from build123d import *

# Parameters (mm, degrees)
SKETCH1_W               = 270
SKETCH1_H               = 100
BOSS_EXTRUDE1_DEPTH     = 3.175
SKETCH1_H_2             = 140
BOSS_EXTRUDE1_2_DEPTH   = 3.175
SKETCH2_R               = 2.5
CUT_EXTRUDE1_DEPTH      = 1
CUT_EXTRUDE1_DEPTH_BACK = 4.175


with BuildPart() as part:
    # Sketch1 → Boss-Extrude1 (new body)
    with BuildSketch(Plane(origin=(0, 0, 0), x_dir=(1, 0, 0), z_dir=(0, 1, 0))):
        with Locations((135, 50)):
            Rectangle(SKETCH1_W, SKETCH1_H)
    extrude(amount=BOSS_EXTRUDE1_DEPTH)


with BuildPart() as body_2:
    # Sketch1 → Boss-Extrude1 2 (new body)
    with BuildSketch(Plane(origin=(0, 0, 0), x_dir=(1, 0, 0), z_dir=(0, 1, 0))):
        with Locations((135, 175)):
            Rectangle(SKETCH1_W, SKETCH1_H_2)
    extrude(amount=BOSS_EXTRUDE1_2_DEPTH)


with BuildPart() as cut_extrude1_tool:
    # Sketch2 → Cut-Extrude1 (new body, two sides)
    with BuildSketch(Plane(origin=(0, 3.175, 0), x_dir=(1, 0, 0), z_dir=(0, 1, 0))) as cut_extrude1_sk:
        with Locations((10, 175)):
            Circle(SKETCH2_R)
        with Locations((10, 50)):
            Circle(SKETCH2_R)
        with Locations((260, 50)):
            Circle(SKETCH2_R)
        with Locations((260, 175)):
            Circle(SKETCH2_R)
        with Locations((135, 115)):
            Circle(SKETCH2_R)
        with Locations((135, 235)):
            Circle(SKETCH2_R)
        with Locations((135, 90)):
            Circle(SKETCH2_R)
        with Locations((135, 10)):
            Circle(SKETCH2_R)
        with BuildLine():
            Line((117.5, 79), (152.5, 79))
            ThreePointArc((152.5, 79), (156.5, 75), (152.5, 71))
            Line((152.5, 71), (117.5, 71))
            ThreePointArc((117.5, 71), (113.5, 75), (117.5, 79))
        make_face()
    extrude(amount=CUT_EXTRUDE1_DEPTH)
    extrude(cut_extrude1_sk.sketch, amount=-CUT_EXTRUDE1_DEPTH_BACK)


with BuildPart() as part_1:
    add(part.part)

    # Cut-Extrude1: cut by cut_extrude1_tool
    add(cut_extrude1_tool.part, mode=Mode.SUBTRACT)


with BuildPart() as body_2_1:
    add(body_2.part)

    # Cut-Extrude1: cut by cut_extrude1_tool
    add(cut_extrude1_tool.part, mode=Mode.SUBTRACT)


solid = part_1.part
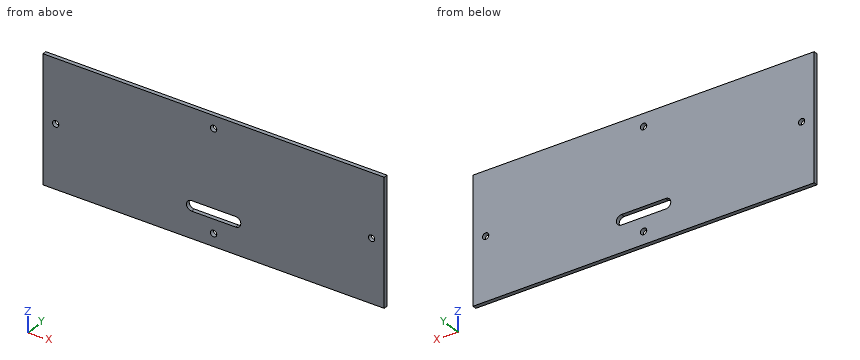
Geometry: final body of the model. Coordinates: model frame, mm. Give positions to 0.01 mm unless a question says otherwise; leave off trailing zeros. Loops run counter-clockwise (first coordinate to the right, second up) from the corner with the lowest first, then second, coordinate; pieces in that order, holes last. Notation, with made-up numbers: (56.5, 51.5) - (114.5, 51.5) arc R9 ccw to (114.5, 62.5) - close; hole circle Ø10 at (-33.5, 78). An arc over 180 degrees is marked (long way). Answer as CSV lines item,"result". Start each with the question number.
1. Ray query, L1, parallel to X at y = 2.25, z = -50; L2, parallel to X at y = 1.1, z = -90; L3, parallel to Z at x = 135, y = 1.65. Return the intervals inside material, ascending.
2. Section B-B, the plane x = 135. Return loops of the section in (y, z) (3 decimals).
3. Section D-D, the plane z = -50. Return loops of the section in (x, y) (3 decimals), plus the area to 4 significant figures.
4. Section C-C, the plane x = 260. Return loops of the section in (y, z) (3 decimals).
5. Pin query (flat end, axial travel): P1, Ø4.5, axis at x = 135, z = -90, coming from the -Y side. Return the tip coordinate at first contact, or that it passes through.
6. Section A-A, the plane z = -10. Return loops of the section in (x, y) (3 decimals), plus the area to 3 significant figures.
Answers:
1,L1,"x = 0 to 7.5, 12.5 to 257.5, 262.5 to 270"
1,L2,"x = 0 to 132.5, 137.5 to 270"
1,L3,"z = -100 to -92.5, -87.5 to -79, -71 to -12.5, -7.5 to 0"
2,outline,"(0, -100) - (3.175, -100) - (3.175, -92.5) - (0, -92.5) - close; (0, -87.5) - (3.175, -87.5) - (3.175, -79) - (0, -79) - close; (0, -71) - (3.175, -71) - (3.175, -12.5) - (0, -12.5) - close; (0, -7.5) - (3.175, -7.5) - (3.175, 0) - (0, 0) - close"
3,outline,"(0, 0) - (7.5, 0) - (7.5, 3.175) - (0, 3.175) - close; (12.5, 0) - (257.5, 0) - (257.5, 3.175) - (12.5, 3.175) - close; (262.5, 0) - (270, 0) - (270, 3.175) - (262.5, 3.175) - close"
3,area,"825.5 mm2"
4,outline,"(0, -100) - (3.175, -100) - (3.175, -52.5) - (0, -52.5) - close; (0, -47.5) - (3.175, -47.5) - (3.175, 0) - (0, 0) - close"
5,P1,"passes through"
6,outline,"(0, 0) - (132.5, 0) - (132.5, 3.175) - (0, 3.175) - close; (137.5, 0) - (270, 0) - (270, 3.175) - (137.5, 3.175) - close"
6,area,"841 mm2"
